Work out the finished part from the listing and answer in its coordinate system (mm). Coordinates: 2 decimals unless noted, no trailing zeros. Order: outer loops, then holes, each group sorted by start corner. A loop starts at its lowest first (then second) coordinate and runs counter-clockwise, first axis right, second up. Notation, with made-up numbers: M 20,-38.5 L 59,-38.5 A26 cw 59,-3.5 Z; hole C 78.5,-23 d7. An arc over 180 degrees is marked long. Answer in a Markdown table with one row per item. Add a question column.
Item 1: Consider line 1 (X direction, y = -4, z = 7.5); line 2 (Z direction, x = -96, y = -9); line 3 (Z direction, x = 10.5, y = -2.5) (1 decimal). Determine where each line is inside the solid, lowest interval first. Write a range as from..to.
Item 2: The part is cut by section C-C (z = -139.5). Write down the section's boundary in (x, y), then the cut area to 3 significant figures.
Item 3: Flat-ended cylindrical pins translate along their axes: pin 1 Ø10 at (x, y) = (-200.5, -8) entering from +Z; pin 2 Ø8 at (y, z) = (-5.5, -147.5) entering from +X; pin 3 Ø3 at (y, z) = (2.5, -197) entering from -X; pin 4 Ø10 at (x, y) = (-137, -4) entering from +Z. Find the tip coordinate at first contact, or state that the pin passes through.
Item 4: The part is cut by section B-B (x = 113.5). Write down the section's boundary in (y, z).
Item 5: The part is cut by section A-A (y = -7). State how many separate pieces and enclosed holes the cut face has, then the cut area to 3 significant figures.
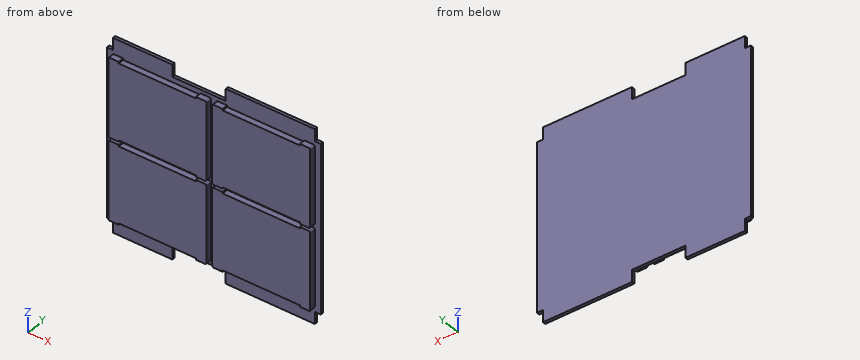
from build123d import *

# Parameters (mm, degrees)
BOSS_EXTRUDE1_DEPTH = 6.35
BOSS_EXTRUDE2_DEPTH = 12.7
FILLET1_R           = 2.54


with BuildPart() as part:
    # Sketch1 → Boss-Extrude1 (new body)
    with BuildSketch(Plane(origin=(0, 0, 0), x_dir=(1, 0, 0), z_dir=(0, 1, 0))):
        Polygon((-228.6, 177.8), (-228.6, -177.8), (-215.9, -177.8), (-215.9, -203.2), (-88.9, -203.2), (-88.9, -177.8), (25.4, -177.8), (25.4, -203.2), (215.9, -203.2), (215.9, -177.8), (228.6, -177.8), (228.6, 177.8), (215.9, 177.8), (215.9, 203.2), (25.4, 203.2), (25.4, 177.8), (-88.9, 177.8), (-88.9, 203.2), (-215.9, 203.2), (-215.9, 177.8), align=None)
    extrude(amount=BOSS_EXTRUDE1_DEPTH)

    # Sketch2 → Boss-Extrude2 (add)
    with BuildSketch(Plane.XZ):
        Polygon((-193.675, 3.17500545), (-193.675, 6.35000545), (-28.575, 6.35000545), (-28.575, 3.17500545), (-6.35, 3.174999665), (-6.35, 169.862499665), (-28.575, 169.862500389), (-28.575, 166.687500389), (-193.675, 166.687500389), (-193.675, 169.862500389), (-215.9, 169.8625), (-215.9, 3.175), align=None)
        Polygon((-6.35, -3.174999665), (-6.35, -169.862499665), (-28.575, -169.862500389), (-28.575, -166.687500389), (-193.675, -166.687500389), (-193.675, -169.862500389), (-215.9, -169.8625), (-215.9, -3.175), (-193.675, -3.17500545), (-193.675, -6.35000545), (-28.575, -6.35000545), (-28.575, -3.17500545), align=None)
        Polygon((193.675, -3.17500545), (193.675, -6.35000545), (28.575, -6.35000545), (28.575, -3.17500545), (6.35, -3.174999665), (6.35, -169.862499665), (28.575, -169.862500389), (28.575, -166.687500389), (193.675, -166.687500389), (193.675, -169.862500389), (215.9, -169.8625), (215.9, -3.175), align=None)
        Polygon((6.35, 3.174999665), (6.35, 169.862499665), (28.575, 169.862500389), (28.575, 166.687500389), (193.675, 166.687500389), (193.675, 169.862500389), (215.9, 169.8625), (215.9, 3.175), (193.675, 3.17500545), (193.675, 6.35000545), (28.575, 6.35000545), (28.575, 3.17500545), align=None)
    extrude(amount=BOSS_EXTRUDE2_DEPTH)

    # Fillet1
    fillet1_edges = [part.edges().sort_by_distance(p)[0] for p in [
        (215.9, -6.35, -169.8625),
        (215.9, -6.35, -3.175),
        (6.35, -6.35, -3.174999665),
        (6.35, -6.35, -169.862499665),
        (-215.9, -6.35, 169.8625),
        (-215.9, -6.35, 3.175),
        (-6.35, -6.35, 3.174999665),
        (-6.35, -6.35, 169.862499665),
        (215.9, -6.35, 169.8625),
        (6.35, -6.35, 169.862499665),
        (6.35, -6.35, 3.174999665),
        (215.9, -6.35, 3.175),
        (-215.9, -6.35, -169.8625),
        (-6.35, -6.35, -169.862499665),
        (-6.35, -6.35, -3.174999665),
        (-215.9, -6.35, -3.175),
    ]]
    fillet(fillet1_edges, radius=FILLET1_R)


solid = part.part
Reply:
| question | item | result |
|---|---|---|
| 1 | line 1 | x = -215.9..-6.35, 6.35..215.9 |
| 1 | line 2 | z = -166.69..-6.35, 6.35..166.69 |
| 1 | line 3 | z = -169.9..-3.2, 3.2..169.9 |
| 2 | outline | M -228.6,0 L -215.9,0 L -215.9,-12.7 L -6.35,-12.7 L -6.35,0 L 6.35,0 L 6.35,-12.7 L 215.9,-12.7 L 215.9,0 L 228.6,0 L 228.6,6.35 L -228.6,6.35 Z |
| 2 | area | 8,230 mm2 |
| 3 | pin 1 | stops at z = 169.86 |
| 3 | pin 2 | stops at x = 215.9 |
| 3 | pin 3 | stops at x = -215.9 |
| 3 | pin 4 | stops at z = 203.2 |
| 4 | outline | M -12.7,-166.69 L 0,-166.69 L 0,-203.2 L 6.35,-203.2 L 6.35,203.2 L 0,203.2 L 0,166.69 L -12.7,166.69 L -12.7,6.35 L 0,6.35 L 0,-6.35 L -12.7,-6.35 Z |
| 5 | separate pieces | 4 |
| 5 | enclosed holes | 0 |
| 5 | area | 136,000 mm2 |
